```python
from build123d import *

# Parameters (mm, degrees)
PINSBASEEXTRUDE_DEPTH      = 0.2
PINSBASEEXTRUDE_DEPTH_BACK = 0.2
PINSBASESKETCH_R           = 28
PINSEXTRUDE_START          = -0.2
PINSSKETCH_R               = 3
PINSEXTRUDE_DEPTH          = 4.4
PINSPATTERN_COUNT          = 10
BOREREVOLVESKETCH_W        = 4
BOREREVOLVESKETCH_H        = 7.5


with BuildPart() as part:
    # PinsBaseSketch → PinsBaseExtrude (new, two sides: drawn at the far end of the back side and taken through both)
    with BuildSketch(Plane.XY.offset(-PINSBASEEXTRUDE_DEPTH_BACK)):
        Circle(PINSBASESKETCH_R)
    extrude(amount=PINSBASEEXTRUDE_DEPTH + PINSBASEEXTRUDE_DEPTH_BACK)

    # PinsSketch → PinsExtrude (add)
    with BuildSketch(Plane.XY.offset(PINSEXTRUDE_START)):
        with Locations((25, 0)):
            Circle(PINSSKETCH_R)
    pinsextrude = extrude(amount=PINSEXTRUDE_DEPTH)

    # PinsPattern: PinsExtrude ×10 about axis
    pinspattern_axis = Axis((0, 0, 0), (0, 0, 1))
    for i in range(1, PINSPATTERN_COUNT):
        add(pinsextrude.rotate(pinspattern_axis, i * 360 / PINSPATTERN_COUNT))

    # BoreRevolveSketch → BoreRevolveCut (revolve, cut)
    with BuildSketch(Plane(origin=(0, 0, 0), x_dir=(0, 0, -1), z_dir=(1, 0, 0)), mode=Mode.PRIVATE) as borerevolvecut_sk:
        with Locations((0, 3.75)):
            Rectangle(BOREREVOLVESKETCH_W, BOREREVOLVESKETCH_H)
    revolve(borerevolvecut_sk.sketch.rotate(Axis((0, 0, 0), (0, 0, -1)), 90), axis=Axis((0, 0, 0), (0, 0, -1)), mode=Mode.SUBTRACT)


solid = part.part
```
Check sheet for the modelled part. Datum: model origin and axes. Units: mm. A direction names the side the tool comes from. Coordinates: 2 decimals unless noted, no trailing zeros. Order: outer loops, then holes, each group sorted by start corner. A loop starts at its lowest first (then second) coordinate and runs counter-clockwise, first axis right, second up. Notation, with made-up numbers: M 8,-38 L 57,-38 A18 cw 57,-15 Z; hole C 59.25,31 d10. An arc over 180 degrees is marked long. Write each question's results on one line, items separated by ' | '. Start each with the question number.
1. Material ranges on probe 1 along Y at (x, z) = (0, 0.15); probe 2 along Y at (x, z) = (20, 2.3); probe 3 along Z at (x, y) = (-21, 0.5), recorded low to high.
2. Cross-section at C-C on y = -5. Record the cut outline in (x, z), and give its area (3 significant figures).
3. Access from +Z, -Z, +X, -X, +Y, -Y to the whole of each face (thin tool, end or side, straight path). Record for faces 1 (the face through (20, 15, 4.2)), 2 (the face through (6, -6, 0.2)).
4. Mould release check, pull along Y, two halves, no side actions. Record for faces 3 (the face through (17.723, 13.04, 2.172)), 4 (the face through (25.865, -10.724, -0.003)), 5 (the face through (-20, -15, 4.2)): +Y half, -Y half, draft (parallel to the pull), parting line (faces both ways), or undercut.
5. Cross-section at B-B on z = 2.8. State how many separate pieces and enclosed holes the cut face has, and give its area (3 significant figures).
6. Cross-section at A-A on x = 0. Record the cut outline in (y, z).
7. Go/stop test with flat-tipped pins: P1, Ø12, axis at x = 1.5, y = 5, coming from the -Z side; P2, Ø17, axis at x = -3.5, y = -1, coming from the +Z side. Record where each tip stops, or that it passes through.
8. Cross-section at D-D on x = 19. Record the cut outline in (y, z), and give its area (3 significant figures).
Checks:
1) probe 1: y = -28 to -7.5, 7.5 to 28 | probe 2: y = -17.69 to -11.7, 11.7 to 17.69 | probe 3: z = -0.2 to 0.2
2) outline: M -27.55,-0.2 L -5.59,-0.2 L -5.59,0.2 L -27.55,0.2 Z; M 5.59,-0.2 L 27.55,-0.2 L 27.55,0.2 L 5.59,0.2 Z | area: 17.6 mm²
3) face 1: +Z, +X, -X, +Y, -Y | face 2: +Z
4) face 3: undercut | face 4: parting line | face 5: draft
5) separate pieces: 10 | enclosed holes: 0 | area: 283 mm²
6) outline: M -28,-0.2 L -7.5,-0.2 L -7.5,0.2 L -28,0.2 Z; M 7.5,-0.2 L 28,-0.2 L 28,0.2 L 7.5,0.2 Z
7) P1: stops at z = -0.2 | P2: stops at z = 0.2
8) outline: M -20.57,-0.2 L 20.57,-0.2 L 20.57,0.2 L 17.43,0.2 L 17.43,4.2 L 11.96,4.2 L 11.96,0.2 L -11.96,0.2 L -11.96,4.2 L -17.43,4.2 L -17.43,0.2 L -20.57,0.2 Z | area: 60.3 mm²
